```python
from build123d import *

# Parameters (mm, degrees)
SKETCH1_W                = 72
SKETCH1_H                = 72
BOSS_EXTRUDE1_DEPTH      = 185
SKETCH2_R                = 15
BOSS_EXTRUDE2_DEPTH      = 20
BOSS_EXTRUDE2_DEPTH_BACK = 205


with BuildPart() as part:
    # Sketch1 → Boss-Extrude1 (new body)
    with BuildSketch(Plane(origin=(0, 0, 0), x_dir=(1, 0, 0), z_dir=(0, 1, 0))):
        Rectangle(SKETCH1_W, SKETCH1_H)
    extrude(amount=BOSS_EXTRUDE1_DEPTH)

    # Sketch2 → Boss-Extrude2 (add, two sides)
    with BuildSketch(Plane(origin=(0, 185, 0), x_dir=(1, 0, 0), z_dir=(0, 1, 0))) as boss_extrude2_sk:
        Circle(SKETCH2_R)
    extrude(amount=BOSS_EXTRUDE2_DEPTH)
    extrude(boss_extrude2_sk.sketch, amount=-BOSS_EXTRUDE2_DEPTH_BACK)


solid = part.part
```
For this review, take the finished solid that the model builds, in its own axes (mm). A direction names the side the tool comes from. Give positions to 0.01 mm unless a question says otherwise; leave off trailing zeros. Write each loop counter-clockwise with the first axis right and the second up, starting at its lowest first coordinate (ties: lowest second). Pieces come first, ordered by that corner, then holes. Notation, with made-up numbers: M 37,-21 L 79,-21 A20 cw 79,1 Z; hole C 68,-10 d6. An arc over 180 degrees is marked long. Answer as a JSON object with one key per item and string values. Group by question number.
Item 1: Consider section D-D on x = 23.5. Write out the cut boundary in (y, z).
Item 2: For pin 1 Ø10 at (x, z) = (20.5, 17) entering from +Y; pin 2 Ø10 at (x, z) = (23, -2.5) entering from -Y, all flat-tipped, find the tip position at first contact; note any pin that passes through.
Item 3: Consider section A-A on x = 0. Write out the cut boundary in (y, z), plus the area to 3 significant figures.
Item 4: Consider section C-C on y = 191. Write out the cut boundary in (x, z), plus the area to 3 significant figures.
Item 5: For probe 1 along Y at (x, z) = (25, 29.5), list the stretches that pass through material, from the lowest coordinate up. Write a range as [from, to].
Item 6: Tool access review of faces 1 (the flat face through (-17, 185, -1)), 2 (the cylindrical face through (-14.985, -9.86, -0.66)), 3 (the flat face through (0, -20, 0)): name each direction out of +Z, -Z, +X, -X, +Y, -Y from which nothing blocks a thin tool from reaching the whole face with its end or side.
Item 7: Consider section B-B on z = 0. Write out the cut boundary in (x, y).
Check result:
{
 "1": {"outline": "M 0,-36 L 185,-36 L 185,36 L 0,36 Z"},
 "2": {"pin 1": "stops at y = 185", "pin 2": "stops at y = 0"},
 "3": {"outline": "M -20,-15 L 0,-15 L 0,-36 L 185,-36 L 185,-15 L 205,-15 L 205,15 L 185,15 L 185,36 L 0,36 L 0,15 L -20,15 Z", "area": "14,500 mm^2"},
 "4": {"outline": "C 0,0 d30", "area": "707 mm^2"},
 "5": {"probe 1": "y = [0, 185]"},
 "6": {"face 1": "+Y", "face 2": "-Y", "face 3": "+Z, -Z, +X, -X, -Y"},
 "7": {"outline": "M -36,0 L -15,0 L -15,-20 L 15,-20 L 15,0 L 36,0 L 36,185 L 15,185 L 15,205 L -15,205 L -15,185 L -36,185 Z"}
}
